```python
from build123d import *

# Parameters (mm, degrees)
F0_W     = 47.70783
F0_H     = 9.607826
F1_DEPTH = 7.8486
F2_R     = 3.0353
F3_DEPTH = 0.889
F4_R     = 3.0353
F5_DEPTH = 0.889
F6_R     = 2.4003
F7_DEPTH = 7.8496
F8_R     = 2.4638
F9_DEPTH = 1.905


with BuildPart() as f1:
    # F0 (on Front) → F1 (new body)
    with BuildSketch(Plane.XZ):
        with Locations((-6.626086, 10.933043)):
            Rectangle(F0_W, F0_H)
    extrude(amount=F1_DEPTH)

    # F2 (on face) → F3 (cut)
    with BuildSketch(Plane.XZ.offset(7.8486)):
        with Locations((-22.618701, 11.939656)):
            Circle(F2_R)
        with Locations((-14.643101, 11.939656)):
            Circle(F2_R)
        with Locations((-6.667501, 11.939656)):
            Circle(F2_R)
        with Locations((1.308099, 11.939656)):
            Circle(F2_R)
        with Locations((9.283699, 11.939656)):
            Circle(F2_R)
    extrude(amount=-F3_DEPTH, mode=Mode.SUBTRACT)

    # F4 (on face) → F5 (cut)
    with BuildSketch(Plane(origin=(0, 0, 0), x_dir=(-1, 0, 0), z_dir=(0, 1, 0))):
        with Locations((-9.239529, 11.939656)):
            Circle(F4_R)
        with Locations((-1.263929, 11.939656)):
            Circle(F4_R)
        with Locations((6.711671, 11.939656)):
            Circle(F4_R)
        with Locations((14.687271, 11.939656)):
            Circle(F4_R)
        with Locations((22.662871, 11.939656)):
            Circle(F4_R)
    extrude(amount=-F5_DEPTH, mode=Mode.SUBTRACT)

    # F6 (on face) → F7 (cut, through all)
    with BuildSketch(Plane.XZ.offset(7.8486)):
        with Locations((-22.618701, 11.939656)):
            Circle(F6_R)
        with Locations((-14.643101, 11.939656)):
            Circle(F6_R)
        with Locations((-6.667501, 11.939656)):
            Circle(F6_R)
        with Locations((1.308099, 11.939656)):
            Circle(F6_R)
        with Locations((9.283699, 11.939656)):
            Circle(F6_R)
    extrude(amount=-F7_DEPTH, mode=Mode.SUBTRACT)

    # F8 (on face) → F9 (join)
    with BuildSketch(Plane.XY.offset(15.736956)):
        with Locations((-26.819086, -3.9243)):
            Circle(F8_R)
        with Locations((-18.741886, -3.9243)):
            Circle(F8_R)
        with Locations((-10.664686, -3.9243)):
            Circle(F8_R)
        with Locations((-2.587486, -3.9243)):
            Circle(F8_R)
        with Locations((5.489714, -3.9243)):
            Circle(F8_R)
        with Locations((13.566914, -3.9243)):
            Circle(F8_R)
    extrude(amount=F9_DEPTH)


solid = f1.part
```
Check sheet for the modelled part. Datum: model origin and axes. Units: mm. A direction names the side the tool comes from. Round coordinates to 2 decimals unless told otherwise and drop trailing zeros. Loops run counter-clockwise (first coordinate to the right, second up) from the corner with the lowest first, then second, coordinate; pieces in that order, holes last. Notation, with made-up numbers: (-26, 76) -> (-8, 76) arc R31 ccw to (-8, 105) -> close; hole circle Ø10 at (51.5, -5). An arc over 180 degrees is marked (long way). Answer in a Markdown table with one row per item.
Q1. Sectioned sample at A-A on x = -23. Enter the section's corners in (y, z), then the cut area to 3 significant figures.
Data:
| item | result |
|---|---|
| outline | (-7.85, 6.13) -> (0, 6.13) -> (0, 8.92) -> (-0.89, 8.92) -> (-0.89, 9.57) -> (-6.96, 9.57) -> (-6.96, 8.93) -> (-7.85, 8.93) -> close; (-7.85, 14.95) -> (-6.96, 14.95) -> (-6.96, 14.31) -> (-0.89, 14.31) -> (-0.89, 14.96) -> (0, 14.96) -> (0, 15.74) -> (-7.85, 15.74) -> close |
| area | 35.9 mm^2 |
Q2. Sectioned sample at B-B on y = -3. Give the number of separate pieces and of enclosed holes in the cut face, then the cut area to 3 significant figures.
Data:
| item | result |
|---|---|
| separate pieces | 1 |
| enclosed holes | 5 |
| area | 420 mm^2 |
Q3. Set-up check for faces 4 (the face through (-0.24, -3.18, 16.68)), 5 (the face through (1.922, -0.438, 8.977)), 6 (the face through (7.515, -3.967, 13.562)), 7 (the face through (-30.48, -4, 11)), 8 (the face through (0.65, -7.41, 8.977)): record each of +Z, -Z, +X, -X, +Y, -Y from which the full face is reachable in a straight line by a thin tool's end or side.
Data:
| item | result |
|---|---|
| face 4 | +Z |
| face 5 | +Y |
| face 6 | +Y, -Y |
| face 7 | +Z, -Z, -X, +Y, -Y |
| face 8 | -Y |
Q4. Thickness scan on L1, parallel to X at y = -1, z = 12; L2, parallel to X at y = -1.5, z = 11.75; L3, parallel to Z at x = 8.5, y = -6. Record the ranges inside material, lowest first.
Data:
| item | result |
|---|---|
| L1 | x = -30.48 to -25.02, -20.22 to -17.04, -12.24 to -9.07, -4.27 to -1.09, 3.71 to 6.88, 11.68 to 17.23 |
| L2 | x = -30.48 to -25.01, -20.23 to -17.04, -12.25 to -9.06, -4.27 to -1.08, 3.7 to 6.89, 11.68 to 17.23 |
| L3 | z = 6.13 to 9.67, 14.21 to 15.74 |
Q5. Release check for a two-part mould opening along Z. For faces 1 (the face through (-8.315, -3.184, 16.676)), 2 (the face through (-6.054, -0.438, 8.977)), 3 (the face through (5, -4, 17.642)) record: released by +Z, released by -Z, zero draft, split by the parting line, or undercut.
Data:
| item | result |
|---|---|
| face 1 | zero draft |
| face 2 | undercut |
| face 3 | released by +Z |
Q6. Go/stop test with flat-tipped pins: P1, Ø1.8, axis at x = 2, z = 11.5, coming from the -Y side; P2, Ø5.5, axis at x = 9.28, z = 11.94, coming from the -Y side; P3, Ø1, axis at x = -24, y = -7, coming from the +Z side; P4, Ø3, axis at x = 8.5, z = 13, coming from the +Y side. Record where each tip stops, or that it passes through.
Data:
| item | result |
|---|---|
| P1 | passes through |
| P2 | stops at y = -6.96 |
| P3 | stops at z = 15.74 |
| P4 | stops at y = -0.89 |
